Part model, mm, in its own coordinate system. Coordinates: 2 decimals unless noted, no trailing zeros. Order: outer loops, then holes, each group sorted by start corner. A loop starts at its lowest first (then second) coordinate and runs counter-clockwise, first axis right, second up. Notation, with made-up numbers: M 67,78.25 L 100,78.25 A34 cw 100,114.25 Z; hole C -12.5,61.5 d10. An arc over 180 degrees is marked long. Answer in a Markdown table with one row per item. Add a question column.
from build123d import *

# Parameters (mm, degrees)
SKETCH007_R      = 4
EXTRUDE008_DEPTH = 2
SKETCH006_R      = 1.2
EXTRUDE006_DEPTH = 2
SKETCH003_R      = 2
EXTRUDE003_DEPTH = 2
SKETCH002_R      = 1.6
SKETCH002_R_2    = 1.2
EXTRUDE002_DEPTH = 2
EXTRUDE_DEPTH    = 2


with BuildPart() as extrude008:
    # Sketch007 → Extrude008 (new body)
    with BuildSketch(Plane.XY):
        with Locations((55, 27)):
            Circle(SKETCH007_R)
    extrude(amount=EXTRUDE008_DEPTH)


with BuildPart() as extrude006:
    # Sketch006 → Extrude006 (new body)
    with BuildSketch(Plane.XY):
        with Locations((11, 11)):
            Circle(SKETCH006_R)
        with Locations((29, 11)):
            Circle(SKETCH006_R)
        with Locations((11, 43)):
            Circle(SKETCH006_R)
        with Locations((29, 43)):
            Circle(SKETCH006_R)
    extrude(amount=EXTRUDE006_DEPTH)


with BuildPart() as extrude003:
    # Sketch003 → Extrude003 (new body)
    with BuildSketch(Plane.XY):
        with Locations((92, 7)):
            Circle(SKETCH003_R)
        with Locations((92, 47)):
            Circle(SKETCH003_R)
    extrude(amount=EXTRUDE003_DEPTH)


with BuildPart() as extrude002:
    # Sketch002 → Extrude002 (new body)
    with BuildSketch(Plane.XY):
        with Locations((5, 5)):
            Circle(SKETCH002_R)
        with Locations((49, 5)):
            Circle(SKETCH002_R)
        with Locations((5, 49)):
            Circle(SKETCH002_R)
        with Locations((49, 49)):
            Circle(SKETCH002_R)
        with Locations((45, 49)):
            Circle(SKETCH002_R_2)
        with Locations((9, 49)):
            Circle(SKETCH002_R_2)
        with Locations((45, 5)):
            Circle(SKETCH002_R_2)
        with Locations((9, 5)):
            Circle(SKETCH002_R_2)
        with Locations((49, 45)):
            Circle(SKETCH002_R_2)
        with Locations((5, 45)):
            Circle(SKETCH002_R_2)
        with Locations((5, 9)):
            Circle(SKETCH002_R_2)
        with Locations((49, 9)):
            Circle(SKETCH002_R_2)
    extrude(amount=EXTRUDE002_DEPTH)


with BuildPart() as part_mirroring001:
    # Part__Mirroring001: instance of Extrude002
    add(extrude002.part.mirror(Plane(origin=(55, 0, 0), x_dir=(0, -1, 0), z_dir=(1, 0, 0))))


with BuildPart() as fusion001:
    # Fusion001 base: copy of Extrude002
    add(extrude002.part)

    # Fusion001: union Part__Mirroring001
    add(part_mirroring001.part)


with BuildPart() as cut004:
    # Sketch → Extrude (new body)
    with BuildSketch(Plane.XY):
        with BuildLine():
            Line((3, 54), (107, 54))
            ThreePointArc((110, 51), (109.12132, 53.12132), (107, 54))
            Line((110, 51), (110, 3))
            ThreePointArc((107, 0), (109.12132, 0.87868), (110, 3))
            Line((107, 0), (3, 0))
            ThreePointArc((0, 3), (0.87868, 0.87868), (3, 0))
            Line((0, 3), (0, 51))
            ThreePointArc((3, 54), (0.87868, 53.12132), (0, 51))
        make_face()
    extrude(amount=EXTRUDE_DEPTH)

    # Cut001: cut Fusion001
    add(fusion001.part, mode=Mode.SUBTRACT)

    # Cut002: cut Extrude003
    add(extrude003.part, mode=Mode.SUBTRACT)

    # Cut003: cut Extrude006
    add(extrude006.part, mode=Mode.SUBTRACT)

    # Cut004: cut Extrude008
    add(extrude008.part, mode=Mode.SUBTRACT)


solid = cut004.part
(1) Slice it at D-D (z = 1.5). State how many separate pieces and enclosed holes the cut face has, and give its area (3 significant figures).
(2) Pull direction Y, two halves, no side cores. Call faces 1 (the cylindrical face through (59.52, 4.39, 0.99)), 2 (the flat face through (54, 54, 1)), 3 (the flat face through (110, 27, 1)): pulls with the +Y half, pulls with the -Y half, needs draft (parallel to the pull), parting line crosses it, or undercut.
(3) Slice it at C-C (x = 55). List the corners of the cut face in (y, z), and give its area (3 significant figures).
(4) Slice it at B-B (y = 27). List the corners of the cut face in (x, z), and give its area (3 significant figures).
(5) Wall check: line 1 (Y direction, x = 11, z = 1.2); line 2 (Y direction, x = 101, z = 1); line 3 (Y direction, x = 60.5, z = 1.9). Give the ranges that are in metal, low to high.
(6) Slice it at A-A (x = 105). List the corners of the cut face in (y, z).
Computed:
| question | item | result |
|---|---|---|
| 1 | separate pieces | 1 |
| 1 | enclosed holes | 31 |
| 1 | area | 5,700 mm^2 |
| 2 | face 1 | undercut |
| 2 | face 2 | pulls with the +Y half |
| 2 | face 3 | needs draft |
| 3 | outline | M 0,0 L 23,0 L 23,2 L 0,2 Z; M 31,0 L 54,0 L 54,2 L 31,2 Z |
| 3 | area | 92.0 mm^2 |
| 4 | outline | M 0,0 L 51,0 L 51,2 L 0,2 Z; M 59,0 L 110,0 L 110,2 L 59,2 Z |
| 4 | area | 204 mm^2 |
| 5 | line 1 | y = 0 to 9.8, 12.2 to 41.8, 44.2 to 54 |
| 5 | line 2 | y = 0 to 3.8, 6.2 to 47.8, 50.2 to 54 |
| 5 | line 3 | y = 0 to 3.48, 6.52 to 7.91, 10.09 to 43.91, 46.09 to 47.48, 50.52 to 54 |
| 6 | outline | M 0,0 L 3.4,0 L 3.4,2 L 0,2 Z; M 6.6,0 L 7.8,0 L 7.8,2 L 6.6,2 Z; M 10.2,0 L 43.8,0 L 43.8,2 L 10.2,2 Z; M 46.2,0 L 47.4,0 L 47.4,2 L 46.2,2 Z; M 50.6,0 L 54,0 L 54,2 L 50.6,2 Z |
